Could you check a few things on this model? Use its own coordinates, in mm. Face numbers are marked on the shaded views. A direction names the side the tool comes from. Give positions to 0.01 mm unless a question says otherwise; leave off trailing zeros. Loops run counter-clockwise (first coordinate to the right, second up) from the corner with the lowest first, then second, coordinate; pieces in that order, holes last. Notation, with made-up numbers: (-20, 60.5) - (25, 60.5) arc R12 ccw to (25, 71.5) - close; hole circle Ø8 at (14.25, 45.25). An arc over 180 degrees is marked (long way). Write each question's results on one line, items separated by ' | '. Start each with the question number.
(1) Suppose I cut it at C-C (x = -43). Please give me the cut outline in (y, z).
(2) On a 3-axis mill with a long thin cutter (end or side, diameter ignored), from which of +Z, -Z, +X, -X, +Y, -Y can I reach the whole of each face in a straight line? I mean the marked faces 1 and 2. Say none if no direction works.
(3) I need wall thicknesses on line 1 (Z direction, x = 0, y = 3.1); line 2 (Y direction, x = 20.5, z = 11.5); line 3 (Z direction, x = -34.5, y = 8.5). Which ranges of each line are inside material? Lowest first, please.
(4) Suppose I cut it at B-B (z = 0). Please give me the cut outline in (x, y), and give its area (3 significant figures).
(5) Suppose I cut it at A-A (x = 0). Please give me the cut outline in (y, z), and give its area (3 significant figures).
(6) For pin 1 (1.5 mm diameter, centred on x = -22, y = 7, fed in from -Z); pin 2 (8 mm diameter, centred on x = -35, z = 1.5, fed in from +Y); pin 3 (4 mm diameter, centred on x = 0, z = 0, fed in from -Y), each with a flat end and sliding along its axis, tell me the tip position at first contact or that it passes through.
(7) Suppose I cut it at D-D (y = 1). Please give me the cut outline in (x, z).
from build123d import *

# Parameters (mm, degrees)
SKETCH1_W                                           = 100
SKETCH1_H                                           = 35
BOSS_EXTRUDE1_DEPTH                                 = 5
SKETCH2_W                                           = 100
SKETCH2_H                                           = 5
BOSS_EXTRUDE2_DEPTH                                 = 10
CSK_FOR_1_4_FLAT_HEAD_MACHINE_SCREW_100_D           = 6.7564
CSK_FOR_1_4_FLAT_HEAD_MACHINE_SCREW_100_CSINK_D     = 12.8778
CSK_FOR_1_4_FLAT_HEAD_MACHINE_SCREW_100_CSINK_ANGLE = 100


with BuildPart() as part:
    # Sketch1 → Boss-Extrude1 (new body)
    with BuildSketch(Plane(origin=(0, 0, 0), x_dir=(1, 0, 0), z_dir=(0, 1, 0))):
        Rectangle(SKETCH1_W, SKETCH1_H)
    extrude(amount=BOSS_EXTRUDE1_DEPTH)

    # Sketch2 → Boss-Extrude2 (add)
    with BuildSketch(Plane(origin=(0, 0, 0), x_dir=(1, 0, 0), z_dir=(0, 1, 0))):
        with Locations((0, -20)):
            Rectangle(SKETCH2_W, SKETCH2_H)
    extrude(amount=BOSS_EXTRUDE2_DEPTH)

    # CSK for 1/4 Flat Head Machine Screw (100)1 (through all)
    with Locations(Plane(origin=(0, 0, 0), x_dir=(-1, 0, 0), z_dir=(0, -1, 0))):
        with Locations((0, 0)):
            CounterSinkHole(CSK_FOR_1_4_FLAT_HEAD_MACHINE_SCREW_100_D / 2, CSK_FOR_1_4_FLAT_HEAD_MACHINE_SCREW_100_CSINK_D / 2, counter_sink_angle=CSK_FOR_1_4_FLAT_HEAD_MACHINE_SCREW_100_CSINK_ANGLE)


solid = part.part
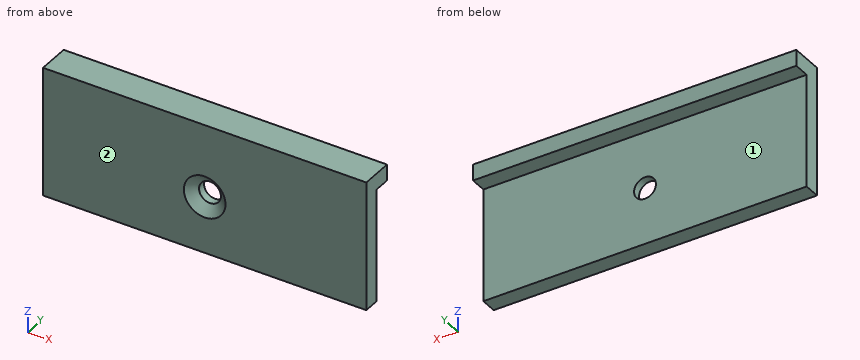
Output values:
1) outline: (0, -17.5) - (5, -17.5) - (5, 17.5) - (10, 17.5) - (10, 22.5) - (0, 22.5) - close
2) face 1: -Z, +X, -X, +Y | face 2: +Z, -Z, +X, -X, -Y
3) line 1: -17.5 to -3.38, 3.38 to 22.5 | line 2: 0 to 5 | line 3: 17.5 to 22.5
4) outline: (-50, 0) - (-6.44, 0) - (-3.38, 2.57) - (-3.38, 5) - (-50, 5) - close; (3.38, 2.57) - (6.44, 0) - (50, 0) - (50, 5) - (3.38, 5) - close | area: 458 mm2
5) outline: (0, -17.5) - (5, -17.5) - (5, -3.38) - (2.57, -3.38) - (0, -6.44) - close; (0, 6.44) - (2.57, 3.38) - (5, 3.38) - (5, 17.5) - (10, 17.5) - (10, 22.5) - (0, 22.5) - close | area: 183 mm2
6) pin 1: z = 17.5 | pin 2: y = 5 | pin 3: through
7) outline: (-50, -17.5) - (50, -17.5) - (50, 22.5) - (-50, 22.5) - close; hole circle Ø10.49 at (0, 0)
